```python
from build123d import *

# Parameters (mm, degrees)
BOSS_EXTRUDE1_DEPTH = 166


with BuildPart() as part:
    # Sketch1 → Boss-Extrude1 (new body)
    with BuildSketch(Plane.XY):
        with BuildLine():
            ThreePointArc((-4.216957229, 111.186498042), (0, 113.5), (4.216957229, 111.186498042))
            Line((4.216957229, 111.186498042), (68.030174337, 11.019811517))
            Line((68.030174337, 11.019811517), (65.5, 9.407912692))
            Line((65.5, 9.407912692), (1.686782892, 109.574599217))
            ThreePointArc((1.686782892, 109.574599217), (0, 110.5), (-1.686782892, 109.574599217))
            Line((-1.686782892, 109.574599217), (-65.5, 9.407912692))
            Line((-65.5, 9.407912692), (-68.030174337, 11.019811517))
            Line((-68.030174337, 11.019811517), (-4.216957229, 111.186498042))
        make_face()
    extrude(amount=BOSS_EXTRUDE1_DEPTH)


solid = part.part
```
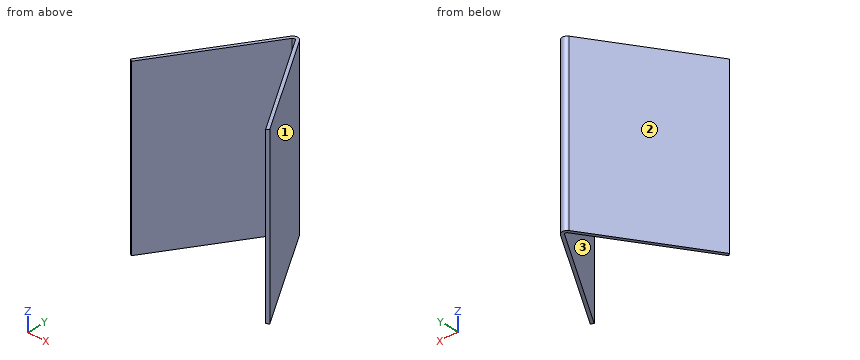
Build history of the part. All positions in model axes, mm. Face numbers are marked on the shaded views. Give positions to 0.01 mm unless a question says otherwise; leave off trailing zeros. Loops run counter-clockwise (first coordinate to the right, second up) from the corner with the lowest first, then second, coordinate; pieces in that order, holes last. Notation, with made-up numbers: (2.5, 83.5) - (46.5, 83.5) arc R20 cw to (46.5, 118.5) - close; hole circle Ø1 at (35.5, 18). An arc over 180 degrees is marked (long way). Use a Markdown table: item, result.
(1) Wall check: line 1 along X through (y, z) = (38, 83.5); line 2 along X through (y, z) = (59.5, 10.5); line 3 along Y through (x, z) = (37, 133). Give the ranges that are in metal, low to high.
Taken from the geometry:
| item | result |
|---|---|
| line 1 | -50.84 to -47.28, 47.28 to 50.84 |
| line 2 | -37.14 to -33.59, 33.59 to 37.14 |
| line 3 | 54.14 to 59.73 |
(2) Band-saw the part on C-C (x = 50.5). Give the cut face in (y, z), and give its area (3 significant figures).
Taken from the geometry:
| item | result |
|---|---|
| outline | (32.95, 0) - (38.54, 0) - (38.54, 166) - (32.95, 166) - close |
| area | 927 mm2 |
(3) Drop flat-ended pins along their axis: pin 1 Ø8 at (x, z) = (-18, 109.5) entering from +Y; pin 2 Ø6 at (x, z) = (-46, 46) entering from +Y; pin 3 Ø1 at (x, z) = (9, 146.5) entering from +Y. Give the stop position or say it passes through.
Taken from the geometry:
| item | result |
|---|---|
| pin 1 | y = 95.83 |
| pin 2 | y = 50.31 |
| pin 3 | y = 104.46 |
(4) Band-saw the part on A-A (y = 42). Give the cut face in (x, z).
Taken from the geometry:
| item | result |
|---|---|
| outline | (-48.29, 0) - (-44.74, 0) - (-44.74, 166) - (-48.29, 166) - close; (44.74, 0) - (48.29, 0) - (48.29, 166) - (44.74, 166) - close |
(5) Band-saw the part on B-B (z = 154). Give the cut face in (x, y), and give its area (3 significant figures).
Taken from the geometry:
| item | result |
|---|---|
| outline | (-68.03, 11.02) - (-65.5, 9.41) - (-1.69, 109.57) arc R2 cw to (1.69, 109.57) - (65.5, 9.41) - (68.03, 11.02) - (4.22, 111.19) arc R5 ccw to (-4.22, 111.19) - close |
| area | 734 mm2 |
(6) Pull direction X, two halves, no side cores. Call the marked faces 1, 2 and 3: +X half, -X half, draft (parallel to the pull), parting line (faces both ways), or undercut.
Taken from the geometry:
| item | result |
|---|---|
| face 1 | +X half |
| face 2 | -X half |
| face 3 | undercut |
